Part print with two shaded views. Sizes in mm from the minimum x, y, z corner. A direction names the side the tool comes from. Round coordinates to 2 decimals unless told otherwise and drop trailing zeros. Loops run counter-clockwise (first coordinate to the right, second up) from the corner with the lowest first, then second, coordinate; pieces in that order, holes last. Notation, with made-up numbers: (58, 57) - (105, 57) arc R16 ccw to (105, 61) - close; hole circle Ø11 at (65, 47). An arc over 180 degrees is marked (long way). Write each question's results on one line, items separated by ' | '. Start each with the question number.
(1) Cut at A-A, the plane z = 6.5. List the corners of the cut face in (x, y), then the cut area to 3 significant figures.
(2) Cut at B-B, the plane x = 15.5. List the corners of the cut face in (y, z).
(3) Mould opens along Y. For the marked faces 1, 2, 3 and 4 say: released by +Y, released by -Y, zero draft, split by the parting line, or undercut.
(4) Cut at C-C, the plane y = 31.5. List the corners of the cut face in (x, z), then the cut area to 3 significant figures.
(5) Flat gauge pins, fed straight in: P1, Ø1.5, axis at x = 10.5, y = 1, coming from the +Z side; P2, Ø6, axis at y = 5, z = 14.5, coming from the +X side; P3, Ø4, axis at x = 19, y = 9.5, coming from the +Z side; P4, Ø6, axis at y = 8, z = 5, coming from the -X side. Where does each tip first touch, or does it go through?
(6) Cut at D-D, the plane z = 11. List the corners of the cut face in (x, y).
(7) Tool access for the marked faces 5 and 6: list every direction of +Z, -Z, +X, -X, +Y, -Y with a clear straight run to the whole face (end or side of a thin tool).
(8) Drill centre lines: L1, parallel to Y at x = 15.25, z = 6; L2, parallel to Y at x = 23.5, z = 3.75. Where is each one in solid material? Low to high.
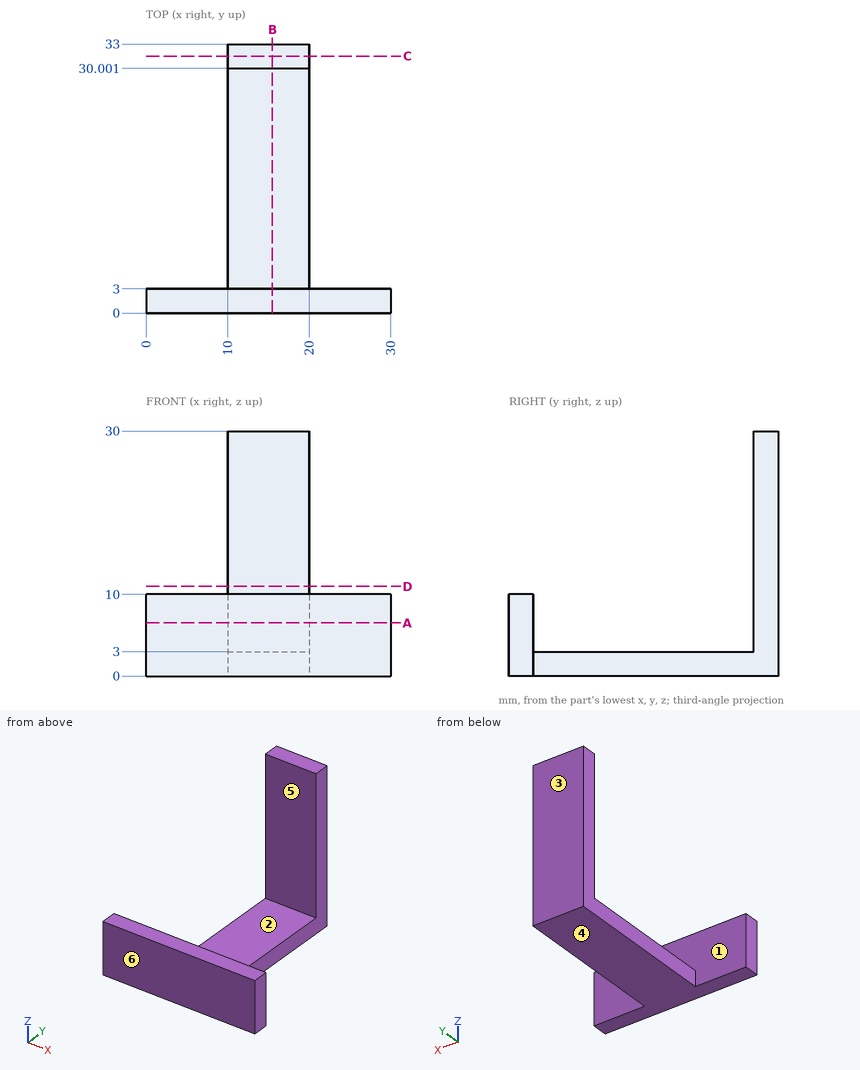
A:
1) outline: (0, 0) - (30, 0) - (30, 3) - (0, 3) - close; (10, 30) - (20, 30) - (20, 33) - (10, 33) - close | area: 120 mm2
2) outline: (0, 0) - (33, 0) - (33, 30) - (30, 30) - (30, 3) - (3, 3) - (3, 10) - (0, 10) - close
3) face 1: undercut | face 2: undercut | face 3: released by +Y | face 4: zero draft
4) outline: (10, 0) - (20, 0) - (20, 30) - (10, 30) - close | area: 300 mm2
5) P1: z = 10 | P2: through | P3: z = 3 | P4: x = 10
6) outline: (10, 30) - (20, 30) - (20, 33) - (10, 33) - close
7) face 5: +Z, +X, -X | face 6: +Z, -Z, +X, -X, -Y
8) L1: 0 to 3, 30 to 33 | L2: 0 to 3
